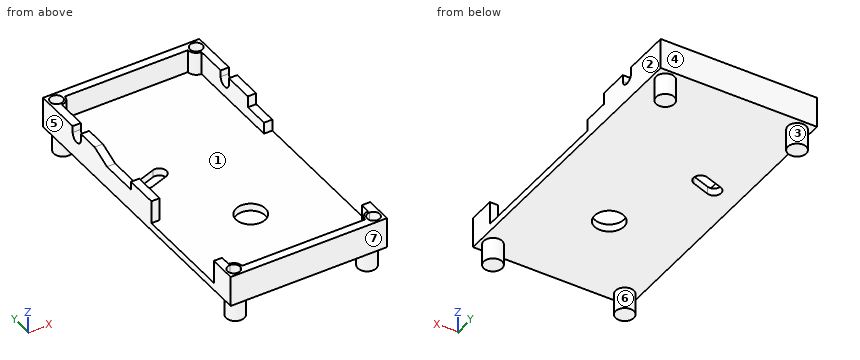
from build123d import *
from build123d.topology import SkipClean

# Parameters (mm, degrees)
SKETCH2_W           = 23.9522
SKETCH2_H           = 45.7962
SKETCH2_R           = 2.2606
BOSS_EXTRUDE1_DEPTH = 4.699
SKETCH4_W           = 21.4122
SKETCH4_H           = 43.2562
CUT_EXTRUDE1_DEPTH  = 3.556
SKETCH5_R           = 1.4097
BOSS_EXTRUDE2_DEPTH = 3.3274
SKETCH6_W           = 3.556
SKETCH6_H           = 15.24
CUT_EXTRUDE3_DEPTH  = 2.54
CUT_EXTRUDE4_DEPTH  = 34.468066413
CUT_EXTRUDE5_DEPTH  = 2.54
BOSS_EXTRUDE3_DEPTH = 3.556
CUT_EXTRUDE6_START  = -3.81
SKETCH12_R          = 0.9652
CUT_EXTRUDE6_DEPTH  = 3.81


with BuildPart() as part:
    # Sketch2 → Boss-Extrude1 (new body)
    with BuildSketch(Plane.XY):
        Rectangle(SKETCH2_W, SKETCH2_H)
        with Locations((0, -8.7249)):
            Circle(SKETCH2_R, mode=Mode.SUBTRACT)
        with BuildLine():
            Line((-8.361518313, 5.139100055), (-5.725634689, 6.065681687))
            ThreePointArc((-5.725634689, 6.065681687), (-4.333034634, 5.3975), (-5.001216321, 4.004899945))
            Line((-5.001216321, 4.004899945), (-7.637099945, 3.078318313))
            ThreePointArc((-7.637099945, 3.078318313), (-9.0297, 3.7465), (-8.361518313, 5.139100055))
        make_face(mode=Mode.SUBTRACT)
    extrude(amount=BOSS_EXTRUDE1_DEPTH)

    # Sketch4 → Cut-Extrude1 (cut)
    with BuildSketch(Plane.XY.offset(4.699)):
        Rectangle(SKETCH4_W, SKETCH4_H)
    extrude(amount=-CUT_EXTRUDE1_DEPTH, mode=Mode.SUBTRACT)

    # Sketch5 → Boss-Extrude2 (add)
    with BuildSketch(Plane(origin=(0, 0, 0), x_dir=(-1, 0, 0), z_dir=(0, 0, -1))):
        with Locations((-10.0965, 21.0185)):
            Circle(SKETCH5_R)
        with Locations(Location((10.0965, 21.0185, 0), (0, 0, 180))):
            Circle(SKETCH5_R)
        with Locations((10.0965, -21.0185)):
            Circle(SKETCH5_R)
        with Locations(Location((-10.0965, -21.0185, 0), (0, 0, 180))):
            Circle(SKETCH5_R)
    extrude(amount=BOSS_EXTRUDE2_DEPTH)

    # Sketch6 → Cut-Extrude3 (cut)
    with BuildSketch(Plane.ZY.offset(11.9761)):
        with Locations((2.921, -11.1633)):
            Rectangle(SKETCH6_W, SKETCH6_H)
        Polygon((4.699, 1.4351), (3.429, 1.4351), (3.429, 7.2771), (4.699, 10.306154579), align=None)
    extrude(amount=-CUT_EXTRUDE3_DEPTH, mode=Mode.SUBTRACT)

    # Sketch6<5> → Cut-Extrude4 (cut, through all)
    with BuildSketch(Plane.ZY.offset(11.9761)):
        with BuildLine():
            Line((3.683, 13.658954579), (4.699, 13.658954579))
            Line((4.699, 13.658954579), (4.699, 15.658954579))
            Line((4.699, 15.658954579), (3.683, 15.658954579))
            ThreePointArc((3.683, 15.658954579), (2.683, 14.658954579), (3.683, 13.658954579))
        make_face()
    extrude(amount=-CUT_EXTRUDE4_DEPTH, mode=Mode.SUBTRACT)

    # Sketch8 → Cut-Extrude5 (cut)
    with BuildSketch(Plane(origin=(11.9761, 0, 0), x_dir=(0, 0, -1), z_dir=(1, 0, 0))):
        Polygon((-4.699, -18.7833), (-1.143, -18.7833), (-1.143, 5.0927), (-2.921, 5.0927), (-2.921, 9.0297), (-4.699, 9.0297), align=None)
    extrude(amount=-CUT_EXTRUDE5_DEPTH, mode=Mode.SUBTRACT)

    # Sketch10 → Boss-Extrude3 (add)
    with BuildSketch(Plane.XY.offset(1.143)):
        with BuildLine():
            Line((-10.7061, 20.6629), (-10.7061, 20.3581))
            ThreePointArc((-10.7061, 20.3581), (-9.808074388, 20.730074388), (-9.4361, 21.6281))
            Line((-9.4361, 21.6281), (-9.7409, 21.6281))
            ThreePointArc((-9.7409, 21.6281), (-10.023600535, 20.945600535), (-10.7061, 20.6629))
        make_face()
        with BuildLine():
            ThreePointArc((9.4361, 21.6281), (9.808074388, 20.730074388), (10.7061, 20.3581))
            Line((10.7061, 20.3581), (10.7061, 20.6629))
            ThreePointArc((10.7061, 20.6629), (10.023600535, 20.945600535), (9.7409, 21.6281))
            Line((9.7409, 21.6281), (9.4361, 21.6281))
        make_face()
        with BuildLine():
            ThreePointArc((-9.4361, -21.6281), (-9.808074388, -20.730074388), (-10.7061, -20.3581))
            Line((-10.7061, -20.3581), (-10.7061, -20.6629))
            ThreePointArc((-10.7061, -20.6629), (-10.023600535, -20.945600535), (-9.7409, -21.6281))
            Line((-9.7409, -21.6281), (-9.4361, -21.6281))
        make_face()
        with BuildLine():
            Line((9.4361, -21.6281), (9.7409, -21.6281))
            ThreePointArc((9.7409, -21.6281), (10.023600535, -20.945600535), (10.7061, -20.6629))
            Line((10.7061, -20.6629), (10.7061, -20.3581))
            ThreePointArc((10.7061, -20.3581), (9.808074388, -20.730074388), (9.4361, -21.6281))
        make_face()
    extrude(amount=BOSS_EXTRUDE3_DEPTH)

    # Sketch12 → Cut-Extrude6 (cut)
    with SkipClean():  # the faces are left unmerged after this step: merging them gives an invalid solid
        with BuildSketch(Plane.XY.offset(4.699).offset(CUT_EXTRUDE6_START)):
            with Locations(Location((-10.7061, 21.6281, 0), (0, 0, 180))):
                Circle(SKETCH12_R)
            with Locations(Location((10.7061, 21.6281, 0), (0, 0, 180))):
                Circle(SKETCH12_R)
            with Locations(Location((10.7061, -21.6281, 0), (0, 0, 180))):
                Circle(SKETCH12_R)
            with Locations(Location((-10.7061, -21.6281, 0), (0, 0, 180))):
                Circle(SKETCH12_R)
        extrude(amount=CUT_EXTRUDE6_DEPTH, mode=Mode.SUBTRACT)


solid = part.part
Design review of the part built by this model. Coordinates are the model's own, in mm. Face numbers are marked on the shaded views. A direction names the side the tool comes from. Coordinates: 2 decimals unless noted, no trailing zeros. Order: outer loops, then holes, each group sorted by start corner. A loop starts at its lowest first (then second) coordinate and runs counter-clockwise, first axis right, second up. Notation, with made-up numbers: M 15,-6.75 L 66,-6.75 A7 ccw 66,6.25 Z; hole C 84.5,-24 d3. An arc over 180 degrees is marked long. Use a Markdown table: item, result.
(1) Add section C-C (x = -3). Give the boundary of the cut face in (y, z), then the cut area to 3 significant figures.
Worked answers:
| item | result |
|---|---|
| outline | M -22.9,0 L 22.9,0 L 22.9,4.7 L 21.63,4.7 L 21.63,1.14 L -21.63,1.14 L -21.63,4.7 L -22.9,4.7 Z |
| area | 61.4 mm2 |
(2) Add section D-D (y = 18). Give the boundary of the cut face in (x, z).
Worked answers:
| item | result |
|---|---|
| outline | M -11.98,0 L 11.98,0 L 11.98,4.7 L 10.71,4.7 L 10.71,1.14 L -10.71,1.14 L -10.71,4.7 L -11.98,4.7 Z |
(3) Wall thickness on probe 1 along Y at (x, z) = (4, 2.5); probe 2 along X at (y, z) = (10, 2.75); probe 3 along Y at (x, z) = (-10.25, 3.25): over which ranges is each line inside the solid? List them lowest first.
Worked answers:
| item | result |
|---|---|
| probe 1 | y = -22.9 to -21.63, 21.63 to 22.9 |
| probe 2 | x = -11.98 to -10.71, 10.71 to 11.98 |
| probe 3 | y = -22.9 to -22.48, -20.78 to -20.44, 20.44 to 20.78, 22.48 to 22.9 |
(4) For the marked faces 1, 2 and 3, list the 3-axis set-ups (+Z, -Z, +X, -X, +Y, -Y) from which the entire face can be reached by the end or side of a thin tool; tool diameter is ignored.
Worked answers:
| item | result |
|---|---|
| face 1 | +Z |
| face 2 | +Z, -Z, +X, +Y, -Y |
| face 3 | -Z |
(5) Draft analysis for pull direction Y (two halves, no side actions). For the marked faces 4, 5, 6 and 7, state which applies: released by +Y, released by -Y, zero draft, split by the parting line, or undercut.
Worked answers:
| item | result |
|---|---|
| face 4 | released by +Y |
| face 5 | zero draft |
| face 6 | undercut |
| face 7 | released by -Y |
(6) Add section B-B (x = 0). Give the boundary of the cut face in (y, z).
Worked answers:
| item | result |
|---|---|
| outline | M -22.9,0 L -10.99,0 L -10.99,1.14 L -21.63,1.14 L -21.63,4.7 L -22.9,4.7 Z; M -6.46,0 L 22.9,0 L 22.9,4.7 L 21.63,4.7 L 21.63,1.14 L -6.46,1.14 Z |
(7) Add section A-A (z = 2). Give the boundary of the cut face in (x, y).
Worked answers:
| item | result |
|---|---|
| outline | M -11.98,-22.9 L 11.98,-22.9 L 11.98,-18.78 L 10.71,-18.78 L 10.71,-20.36 A1.27 ccw 9.44,-21.63 L -9.44,-21.63 A1.27 ccw -10.71,-20.36 L -10.71,-18.78 L -11.98,-18.78 Z; M -11.98,-3.54 L -10.71,-3.54 L -10.71,20.36 A1.27 ccw -9.44,21.63 L 9.44,21.63 A1.27 ccw 10.71,20.36 L 10.71,5.09 L 11.98,5.09 L 11.98,22.9 L -11.98,22.9 Z; hole C -10.71,-21.63 d1.93; hole C -10.71,21.63 d1.93; hole C 10.71,-21.63 d1.93; hole C 10.71,21.63 d1.93 |
(8) For P1, Ø3, axis at x = 3, y = 4, coming from the +Z side; P2, Ø6, axis at x = 0, y = -8.72, coming from the -Z side, all flat-tipped, find the tip position at first contact; note any pin that passes through.
Worked answers:
| item | result |
|---|---|
| P1 | stops at z = 1.14 |
| P2 | stops at z = 0 |
